Here's how the part is built. I have some questions about the finished solid (model axes, mm). Face numbers are marked on the shaded views. A direction names the side the tool comes from. Round coordinates to 2 decimals unless told otherwise and drop trailing zeros. Write each loop counter-clockwise with the first axis right and the second up, starting at its lowest first coordinate (ties: lowest second). Pieces come first, ordered by that corner, then holes. Notation, with made-up numbers: (18.25, -27) - (68.25, -27) arc R20 ccw to (68.25, 7) - close; hole circle Ø1 at (13.5, -30.5). An arc over 180 degrees is marked (long way). Use one line per item in the form item = value. Start each with the question number.
1. I want a section at D-D, the plane z = 3.75. State how many separate pieces and enclosed holes the cut face has, plus the area to 3 significant figures.
2. We'd pull the mould along X, two halves only. Please class the marked faces 1, 2 and 3: +X half, -X half, draft (parallel to the pull), parting line (faces both ways), or undercut.
3. I want a section at C-C, the plane y = 17. List the corners of the cut face in (x, z) for me, plus the area to 3 significant figures.
4. If I drill on line 1 along X through (y, z) = (47, 2.05); line 2 along Y through (x, z) = (43, 4.7); line 3 along X through (y, z) = (22, 1.6), over which ranges is the centre line in solid material (lowest first)?
5. Will these pins go through, and if not, where does the flat tip stop? pin 1 (2 mm diameter, centred on y = 47, z = 1, fed in from -X); pin 2 (1.5 mm diameter, centred on x = 35.5, z = 3.5, fed in from +Y).
6. I want a section at A-A, the plane y = 29. List the corners of the cut face in (x, z) for me.
7. I want a section at B-B, the plane x = 75.5. List the corners of the cut face in (y, z) for me.
8. Which directions (+Z, -Z, +X, -X, +Y, -Y) give clear straight access to the entire face, cutting with the end or side of a thin tool? Please do the marked faces 4, 5, 6, 7 and 8.
```python
from build123d import *

# Parameters (mm, degrees)
MODEL_R                  = 1.8
MODEL_W                  = 6.9
MODEL_H                  = 7.1
RESSALTO_EXTRUS_O1_DEPTH = 6


with BuildPart() as part:
    # Model → Ressalto-extrusão1 (new body)
    with BuildSketch(Plane.XY):
        Polygon((98.034292433, 10.612136161), (98.134192856, 10.370955206), (98.16826703, 10.112136161), (98.16826703, 7.512443376), (98.134192856, 7.25362433), (98.034292433, 7.012443376), (97.875373811, 6.805336594), (97.66826703, 6.646417972), (97.427086075, 6.546517549), (97.16826703, 6.512443376), (34.067480382, 6.516377235), (33.808814837, 6.550620973), (33.567812927, 6.650613857), (33.360882181, 6.809548321), (33.202110548, 7.016604029), (33.102307278, 7.257684523), (33.06826703, 7.516376926), (33.06826703, 10.110713257), (33.102341203, 10.369532302), (33.202241626, 10.610713257), (33.361160249, 10.817820038), (33.56826703, 10.97673866), (33.809447985, 11.076639083), (34.06826703, 11.110713257), (39.06826703, 11.110713257), (39.06826703, 20.610713257), (34.06826703, 20.610713257), (33.809447985, 20.64478743), (33.56826703, 20.744687853), (33.361160249, 20.903606475), (33.202241626, 21.110713257), (33.102341203, 21.351894212), (33.06826703, 21.610713257), (33.06826703, 42.910713257), (33.102341203, 43.169532302), (33.202241626, 43.410713257), (33.361160249, 43.617820038), (33.56826703, 43.77673866), (33.809447985, 43.876639083), (34.06826703, 43.910713257), (39.06826703, 43.910713257), (39.06826703, 55.210713257), (92.16826703, 55.210713257), (92.16826703, 43.910713257), (97.16826703, 43.910713257), (97.427086075, 43.876639083), (97.66826703, 43.77673866), (97.875373811, 43.617820038), (98.034292433, 43.410713257), (98.134192856, 43.169532302), (98.16826703, 42.910713257), (98.16826703, 21.610713257), (98.134192856, 21.351894212), (98.034292433, 21.110713257), (97.875373811, 20.903606475), (97.66826703, 20.744687853), (97.427086075, 20.64478743), (97.16826703, 20.610713257), (92.16826703, 20.610713257), (92.16826703, 11.112136161), (97.16826703, 11.112136161), (97.427086075, 11.078061987), (97.66826703, 10.978161564), (97.875373811, 10.819242942), align=None)
        with Locations((49.16826703, 11.028176846)):
            Circle(MODEL_R, mode=Mode.SUBTRACT)
        with Locations((82.06826703, 11.028176846)):
            Circle(MODEL_R, mode=Mode.SUBTRACT)
        with Locations((88.11826703, 50.210713257)):
            Circle(MODEL_R, mode=Mode.SUBTRACT)
        with Locations((43.11826703, 50.210713257)):
            Circle(MODEL_R, mode=Mode.SUBTRACT)
        with Locations((80.91826703, 46.878174347)):
            Rectangle(MODEL_W, MODEL_H, mode=Mode.SUBTRACT)
        Polygon((53.76826703, 27.328179344), (53.76826703, 19.959715186), (46.86826703, 19.959715186), (46.86826703, 27.328179344), (40.618277181, 27.328179344), (40.618277181, 38.328174347), (90.618256879, 38.328174347), (90.618256879, 27.328179344), (84.36826703, 27.328179344), (84.36826703, 19.959715186), (77.46826703, 19.959715186), (77.46826703, 27.328179344), align=None, mode=Mode.SUBTRACT)
        with Locations((50.31826703, 46.878174347)):
            Rectangle(MODEL_W, MODEL_H, mode=Mode.SUBTRACT)
    extrude(amount=RESSALTO_EXTRUS_O1_DEPTH)


solid = part.part
```
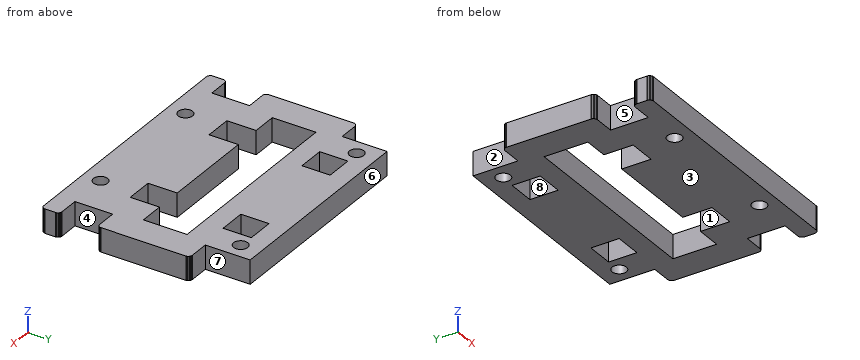
Model answer:
q1.separate_pieces = 1
q1.enclosed_holes = 7
q1.area = 2,130 mm2
q2.face_1 = undercut
q2.face_2 = -X half
q2.face_3 = draft
q3.outline = (39.07, 0) - (92.17, 0) - (92.17, 6) - (39.07, 6) - close
q3.area = 319 mm2
q4.line_1 = 39.07 to 46.87, 53.77 to 77.47, 84.37 to 92.17
q4.line_2 = 6.52 to 27.33, 38.33 to 48.41, 52.01 to 55.21
q4.line_3 = 33.07 to 46.87, 53.77 to 77.47, 84.37 to 98.17
q5.pin_1 = 39.07
q5.pin_2 = 43.91
q6.outline = (33.07, 0) - (40.62, 0) - (40.62, 6) - (33.07, 6) - close; (90.62, 0) - (98.17, 0) - (98.17, 6) - (90.62, 6) - close
q7.outline = (6.51, 0) - (27.33, 0) - (27.33, 6) - (6.51, 6) - close; (38.33, 0) - (55.21, 0) - (55.21, 6) - (38.33, 6) - close
q8.face_4 = +Z, -Z, +X
q8.face_5 = +Z, -Z, -X
q8.face_6 = +Z, -Z, +X, -X, +Y
q8.face_7 = +Z, -Z, +X, +Y
q8.face_8 = +Z, -Z
